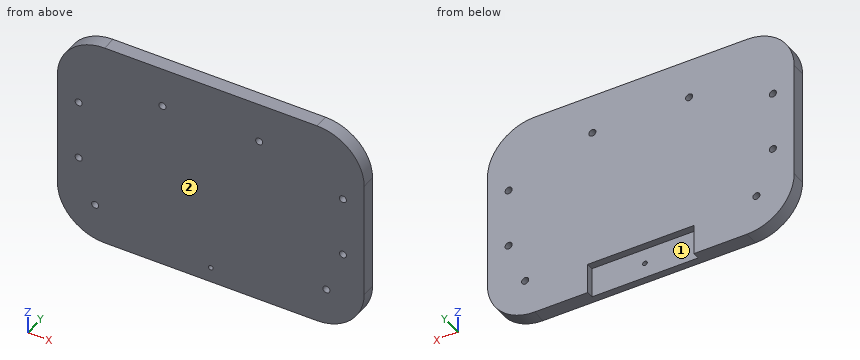
```python
from build123d import *

# Parameters (mm, degrees)
BOSS_EXTRUDE1_DEPTH       = 6
SKETCH3_W                 = 45
SKETCH3_H                 = 13
CUT_EXTRUDE1_DEPTH        = 3
F_2_0MM_DOWEL_HOLE1_D     = 2
F_2_0MM_DOWEL_HOLE1_DEPTH = 12
F_2_0MM_DOWEL_HOLE1_TIP   = 0.600860619
F_3_0MM_DOWEL_HOLE1_D     = 3
F_3_0MM_DOWEL_HOLE1_DEPTH = 12
F_3_0MM_DOWEL_HOLE1_TIP   = 0.901290929


with BuildPart() as part:
    # Sketch2 → Boss-Extrude1 (new body)
    with BuildSketch(Plane(origin=(0, 0, 0), x_dir=(1, 0, 0), z_dir=(0, 1, 0))):
        with BuildLine():
            Line((-20, 0), (-110, 0))
            ThreePointArc((-110, 0), (-124.142135624, 5.857864376), (-130, 20))
            Line((-130, 20), (-130, 70))
            ThreePointArc((-130, 70), (-124.142135624, 84.142135624), (-110, 90))
            Line((-110, 90), (-20, 90))
            ThreePointArc((-20, 90), (-5.857864376, 84.142135624), (0, 70))
            Line((0, 70), (0, 20))
            ThreePointArc((0, 20), (-5.857864376, 5.857864376), (-20, 0))
        make_face()
    extrude(amount=BOSS_EXTRUDE1_DEPTH)

    # Sketch3 → Cut-Extrude1 (cut)
    with BuildSketch(Plane(origin=(0, 6, 0), x_dir=(1, 0, 0), z_dir=(0, 1, 0))):
        with Locations((-65, 83.5)):
            Rectangle(SKETCH3_W, SKETCH3_H)
    extrude(amount=-CUT_EXTRUDE1_DEPTH, mode=Mode.SUBTRACT)

    # Ø2.0mm Dowel Hole1
    with Locations(Plane(origin=(0, 3, 0), x_dir=(1, 0, 0), z_dir=(0, 1, 0))):
        with Locations((-65, 83.5)):
            Hole(F_2_0MM_DOWEL_HOLE1_D / 2, depth=F_2_0MM_DOWEL_HOLE1_DEPTH)
            with Locations((0, 0, -(F_2_0MM_DOWEL_HOLE1_DEPTH + F_2_0MM_DOWEL_HOLE1_TIP / 2))):  # 118° drill point
                Cone(0, F_2_0MM_DOWEL_HOLE1_D / 2, F_2_0MM_DOWEL_HOLE1_TIP, mode=Mode.SUBTRACT)

    # Ø3.0mm Dowel Hole1
    with Locations(Plane(origin=(0, 6, 0), x_dir=(1, 0, 0), z_dir=(0, 1, 0))):
        with Locations((-114, 74), (-16, 74), (-121, 55), (-9, 55), (-121, 29.5), (-9, 29.5), (-85.5, 17), (-44.5, 17)):
            Hole(F_3_0MM_DOWEL_HOLE1_D / 2, depth=F_3_0MM_DOWEL_HOLE1_DEPTH)
            with Locations((0, 0, -(F_3_0MM_DOWEL_HOLE1_DEPTH + F_3_0MM_DOWEL_HOLE1_TIP / 2))):  # 118° drill point
                Cone(0, F_3_0MM_DOWEL_HOLE1_D / 2, F_3_0MM_DOWEL_HOLE1_TIP, mode=Mode.SUBTRACT)


solid = part.part
```
Geometry check sheet. Reference: the model listing, model coordinates, mm. Face numbers are marked on the shaded views. Give positions to 0.01 mm unless a question says otherwise; leave off trailing zeros. Write each loop counter-clockwise with the first axis right and the second up, starting at its lowest first coordinate (ties: lowest second). Pieces come first, ordered by that corner, then holes.
1) Section check C-C, the plane z = -80.5. Record the boundary of the cut face in (x, y).
2) Section check A-A, the plane x = -85.5. Record the boundary of the cut face in (y, z), and give its area (3 significant figures).
3) Section check B-B, the plane z = -29.5. Record the boundary of the cut face in (x, y).
4) Section check D-D, the plane z = -10.5. Record the boundary of the cut face in (x, y), and give its area (3 significant figures).
5) Gauge pin test, flat ends, axial feed: pin 1 (2.5 mm diameter, centred on y = 5, z = -82.5, fed in from +X); pin 2 (3.5 mm diameter, centred on x = -60, y = 5, fed in from -Z); pin 3 (10.5 mm diameter, centred on x = -63.5, z = -84, fed in from +Y). Record the tip position at first contact, or that the pin passes through.
6) Release check for a two-part mould opening along X. For the marked faces 1 and 2 record: pulls with the +X half, pulls with the -X half, needs draft (parallel to the pull), parting line crosses it, or undercut.
7) Material ranges on L1, parallel to X at y = 2.5, z = -29.5; L2, parallel to Z at x = -9, y = 2.85; L3, parallel to X at y = 3.65, z = -17, recorded low to high.
Computed:
1. outline: (-127.02, 0) - (-2.98, 0) - (-2.98, 6) - (-42.5, 6) - (-42.5, 3) - (-87.5, 3) - (-87.5, 6) - (-127.02, 6) - close
2. outline: (0, -90) - (3, -90) - (3, -77) - (6, -77) - (6, -18.5) - (0, -18.5) - close; (0, -15.5) - (6, -15.5) - (6, 0) - (0, 0) - close
2. area: 483 mm2
3. outline: (-130, 0) - (-122.5, 0) - (-122.5, 6) - (-130, 6) - close; (-119.5, 0) - (-10.5, 0) - (-10.5, 6) - (-119.5, 6) - close; (-7.5, 0) - (0, 0) - (0, 6) - (-7.5, 6) - close
4. outline: (-127.6, 0) - (-2.4, 0) - (-2.4, 6) - (-127.6, 6) - close
4. area: 751 mm2
5. pin 1: stops at x = -3.46
5. pin 2: stops at z = -77
5. pin 3: stops at y = 3
6. face 1: undercut
6. face 2: needs draft
7. L1: x = -130 to -122.5, -119.5 to -10.5, -7.5 to 0
7. L2: z = -86.7 to -56.5, -53.5 to -31, -28 to -3.3
7. L3: x = -129.77 to -87, -84 to -46, -43 to -0.23
